Could you check a few things on this model? Use its own coordinates, in mm. Face numbers are marked on the shaded views. Coordinates: 2 decimals unless noted, no trailing zeros. Write each loop counter-clockwise with the first axis right and the second up, starting at its lowest first coordinate (ties: lowest second). Pieces come first, ordered by that corner, then holes.
Item 1: For P1, Ø5, axis at x = -33.5, y = -3.5, coming from the +Z side; P2, Ø1.2, axis at x = -68, z = 6, coming from the +Y side, each with a flat end and sliding along its axis, tell me the tip position at first contact or that it passes through.
Item 2: I want a section at A-A on z = 4.5. Please give me the cut outline in (x, y) (3 decimals).
Item 3: If I drill on probe 1 along X at (y, z) = (6.5, 9.75) (3 decimals); probe 2 along Z at (x, y) = (52, -7.5); probe 3 along X at (y, z) = (-8.75, 4.5), over which ranges is the centre line in solid material (lowest first)?
Item 4: I want a section at B-B on y = 4.25. Please give me the cut outline in (x, z) (3 decimals).
Item 5: Thinking about a two-plate mould opening in X: for the marked faces 1, 2, 3 and 4, which applies, +X half, -X half, draft (parallel to the pull), parting line (faces both ways), or undercut?
Item 6: I want a section at D-D on x = -45.5. Please give me the cut outline in (y, z), then the cut area to 3 significant figures.
Item 7: I want a section at C-C on x = 11.5. Please give me the cut outline in (y, z), then the cut area to 3 significant figures.
from build123d import *

# Parameters (mm, degrees)
EXTRUDE_1_DEPTH = 2
EXTRUDE_2_DEPTH = 15


with BuildPart() as part:
    # 스케치1 → 보스-돌출1 (new body)
    with BuildSketch(Plane.XY):
        Polygon((-69.825, -7), (99.75, -10), (99.75, 10), (-69.825, 7), align=None)
    extrude(amount=EXTRUDE_1_DEPTH)

    # 스케치2 → 보스-돌출2 (add)
    with BuildSketch(Plane.XY.offset(2)):
        Polygon((-65.825, 7), (-69.825, 7), (-69.825, -7), (-65.825, -7.070765148), align=None)
        Polygon((99.75, 10), (95.16, 9.918796992), (95.16, -9.918796992), (99.75, -9.918796992), align=None)
        Polygon((99.75, -9.918796992), (95.16, -9.918796992), (99.75, -10), align=None)
    extrude(amount=EXTRUDE_2_DEPTH)


solid = part.part
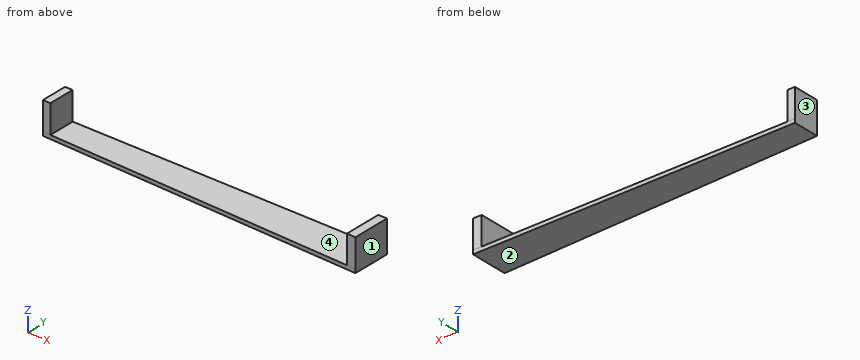
Response values:
1. P1: stops at z = 2
1. P2: stops at y = 7
2. outline: (-69.825, -7) - (-65.825, -7.071) - (-65.825, 7) - (-69.825, 7) - close; (95.16, -9.919) - (99.75, -10) - (99.75, 10) - (95.16, 9.919) - close
3. probe 1: x = -69.825 to -65.825, 95.16 to 99.75
3. probe 2: z = 0 to 2
3. probe 3: x = 95.16 to 99.75
4. outline: (-69.825, 0) - (99.75, 0) - (99.75, 17) - (95.16, 17) - (95.16, 2) - (-65.825, 2) - (-65.825, 17) - (-69.825, 17) - close
5. face 1: +X half
5. face 2: draft
5. face 3: -X half
5. face 4: undercut
6. outline: (-7.43, 0) - (7.43, 0) - (7.43, 2) - (-7.43, 2) - close
6. area: 29.7 mm2
7. outline: (-8.44, 0) - (8.44, 0) - (8.44, 2) - (-8.44, 2) - close
7. area: 33.8 mm2
